from build123d import *

# Parameters (mm, degrees)
CROQUIS1_R              = 55
CROQUIS1_R_2            = 20
SALIENTE_EXTRUIR1_DEPTH = 10
CROQUIS2_R              = 6
CROQUIS2_R_2            = 20
SALIENTE_EXTRUIR2_DEPTH = 20
CROQUIS3_R              = 6
CORTAR_EXTRUIR2_DEPTH   = 81.311892021
CROQUIS4_R              = 4.75
SALIENTE_EXTRUIR3_DEPTH = 5
MATRIZC1_COUNT          = 4
CROQUIS5_R              = 4
CORTAR_EXTRUIR3_DEPTH   = 2.5
MATRIZC2_COUNT          = 6


with BuildPart() as part:
    # Croquis1 → Saliente-Extruir1 (new body)
    with BuildSketch(Plane.XY):
        Circle(CROQUIS1_R)
        Circle(CROQUIS1_R_2, mode=Mode.SUBTRACT)
    extrude(amount=SALIENTE_EXTRUIR1_DEPTH)

    # Croquis2 → Saliente-Extruir2 (add)
    # profile 1 of 7: a face of its own
    with BuildSketch(Plane.XY):
        with Locations((17.368749874, 30.386288484)):
            Circle(CROQUIS2_R)
    # profile 2 of 7: a face of its own
    with BuildSketch(Plane.XY):
        with Locations((35.570236927, 0.06310586)):
            Circle(CROQUIS2_R)
    # profile 3 of 7: a face of its own
    with BuildSketch(Plane.XY):
        with Locations((18.410333978, -30.861435627)):
            Circle(CROQUIS2_R)
    # profile 4 of 7: a face of its own
    with BuildSketch(Plane.XY):
        with Locations((-16.951056024, -31.462794489)):
            Circle(CROQUIS2_R)
    # profile 5 of 7: a face of its own
    with BuildSketch(Plane.XY):
        with Locations((-35.152543077, -1.139611866)):
            Circle(CROQUIS2_R)
    # profile 6 of 7: a face of its own
    with BuildSketch(Plane.XY):
        with Locations((-17.992640128, 29.784929621)):
            Circle(CROQUIS2_R)
    # profile 7 of 7: a face of its own
    with BuildSketch(Plane.XY):
        with BuildLine():
            ThreePointArc((-27.174096814, 22.058296905), (-30.772867756, 16.67424991), (-33.318098438, 10.719343099))
            ThreePointArc((-33.318098438, 10.719343099), (-23.158844078, -0.750787602), (-32.553845663, -12.8548486))
            ThreePointArc((-32.553845663, -12.8548486), (-29.724252158, -18.478875336), (-25.932896476, -23.504996924))
            ThreePointArc((-25.932896476, -23.504996924), (-11.259372102, -20.898480308), (-5.36472656, -34.58640931))
            ThreePointArc((-5.36472656, -34.58640931), (0.788104907, -34.991125884), (6.916475444, -34.309799875))
            ThreePointArc((6.916475444, -34.309799875), (12.262561294, -20.555859902), (26.90508267, -22.385632145))
            ThreePointArc((26.90508267, -22.385632145), (30.429526117, -17.292886986), (33.001146459, -11.658659117))
            ThreePointArc((33.001146459, -11.658659117), (23.570255812, 0.041816456), (32.959571133, 11.775681328))
            ThreePointArc((32.959571133, 11.775681328), (30.28541045, 17.544056369), (26.611824153, 22.733473454))
            ThreePointArc((26.611824153, 22.733473454), (11.413749917, 19.968132432), (6.083961325, 34.467164296))
            ThreePointArc((6.083961325, 34.467164296), (-0.405697858, 34.997648625), (-6.881315891, 34.316868907))
            ThreePointArc((-6.881315891, 34.316868907), (-11.787864219, 19.513573531), (-27.174096814, 22.058296905))
        make_face()
        Circle(CROQUIS2_R_2, mode=Mode.SUBTRACT)
    extrude(amount=SALIENTE_EXTRUIR2_DEPTH)

    # Croquis3 → Cortar-Extruir2 (cut, through all)
    with BuildSketch(Plane.XY.offset(20)):
        with Locations((-17.992640128, 29.784929621)):
            Circle(CROQUIS3_R)
        with Locations((-35.152543077, -1.139611866)):
            Circle(CROQUIS3_R)
        with Locations((-16.951056024, -31.462794489)):
            Circle(CROQUIS3_R)
        with Locations((18.410333978, -30.861435627)):
            Circle(CROQUIS3_R)
        with Locations((35.570236927, 0.06310586)):
            Circle(CROQUIS3_R)
        with Locations((17.368749874, 30.386288484)):
            Circle(CROQUIS3_R)
    extrude(amount=-CORTAR_EXTRUIR2_DEPTH, mode=Mode.SUBTRACT)

    # Croquis4 → Saliente-Extruir3 (add, symmetric)
    with BuildSketch(Plane(origin=(0, 55, 0), x_dir=(1, 0, 0), z_dir=(0, 1, 0))):
        with Locations(Location((0, -5.001814487, 0), (0, 0, 90))):
            Circle(CROQUIS4_R)
    saliente_extruir3 = extrude(amount=SALIENTE_EXTRUIR3_DEPTH, both=True)

    # MatrizC1: Saliente-Extruir3 ×4 about axis
    matrizc1_axis = Axis((0, 0, 0), (0, 0, 1))
    for i in range(1, MATRIZC1_COUNT):
        add(saliente_extruir3.rotate(matrizc1_axis, i * 360 / MATRIZC1_COUNT))

    # Croquis5 → Cortar-Extruir3 (cut, symmetric)
    with BuildSketch(Plane(origin=(0, 35, 0), x_dir=(1, 0, 0), z_dir=(0, 1, 0))):
        with Locations(Location((0, -15.307164254, 0), (0, 0, 270))):
            Circle(CROQUIS5_R)
    cortar_extruir3 = extrude(amount=CORTAR_EXTRUIR3_DEPTH, both=True, mode=Mode.SUBTRACT)

    # MatrizC2: Cortar-Extruir3 ×6 about axis
    matrizc2_axis = Axis((0, 0, 0), (0, 0, 1))
    for i in range(1, MATRIZC2_COUNT):
        add(cortar_extruir3.rotate(matrizc2_axis, i * 360 / MATRIZC2_COUNT), mode=Mode.SUBTRACT)


solid = part.part
Geometry: final body of the model. Coordinates: model frame, mm. A direction names the side the tool comes from. Coordinates: 2 decimals unless noted, no trailing zeros. Order: outer loops, then holes, each group sorted by start corner. A loop starts at its lowest first (then second) coordinate and runs counter-clockwise, first axis right, second up. Notation, with made-up numbers: (64.25, 10) - (78.25, 10) arc R16 cw to (78.25, 34) - close; hole circle Ø1 at (6.25, 30.5). An arc over 180 degrees is marked (long way). Use one line per item in the form item = value.
1) Section B-B (z = 4.5). Return loops of the section in (x, y).
Solutions:
outline = (-60, -4.72) - (-54.8, -4.72) arc R55 ccw to (-4.72, -54.8) - (-4.72, -60) - (4.72, -60) - (4.72, -54.8) arc R55 ccw to (54.8, -4.72) - (60, -4.72) - (60, 4.72) - (54.8, 4.72) arc R55 ccw to (4.72, 54.8) - (4.72, 60) - (-4.72, 60) - (-4.72, 54.8) arc R55 ccw to (-54.8, 4.72) - (-60, 4.72) - close; hole circle Ø12 at (-35.15, -1.14); hole circle Ø12 at (-17.99, 29.78); hole circle Ø12 at (-16.95, -31.46); hole circle Ø40 at (0, 0); hole circle Ø12 at (17.37, 30.39); hole circle Ø12 at (18.41, -30.86); hole circle Ø12 at (35.57, 0.06)
2) Section D-D (x = -45). Return loops of the section in (y, z).
Solutions:
outline = (-31.62, 0) - (31.62, 0) - (31.62, 10) - (-31.62, 10) - close
3) Set-up query: faces 1 (the face through (1.427, -57.433, 0.471)), 2 (the face through (28.118, -16.298, 15.251)), 3 (the face through (57.434, 1.427, 0.471)), 4 (the face through (12.073, -20.672, 14.93)), 5 (the face through (-23.17, -0.52, 14.93)). Return all of +Z, -Z, +X, -X, +Y, -Y with unobstructed straight access to the full face (end or side cutting, diameter ignored); none if empty.
Solutions:
face_1 = -Y
face_2 = none
face_3 = +X
face_4 = +Z
face_5 = +Z, -X
4) Ray query, L1, parallel to X at y = -4.5, z = 8; L2, parallel to Y at x = 0, z = 14; L3, parallel to X at y = 33, z = 8.75. Return the intervals inside material, ascending.
Solutions:
L1 = -54.82 to -40.12, -30.18 to -19.49, 19.49 to 31.67, 39.47 to 54.82
L2 = -32.5 to -20, 20 to 32.5
L3 = -44 to -23.06, -12.93 to 11.97, 22.77 to 44
5) Mould query, pull axis Y, two halves, no side actions, for faces 6 (the face through (-57.434, -1.427, 0.471)), 7 (the face through (32.22, 13.67, 14.93)), 8 (the face through (29.33, 16.73, 11.31)). Classes: +Y half, -Y half, draft (parallel to the pull), parting line (faces both ways), or undercut.
Solutions:
face_6 = parting line
face_7 = +Y half
face_8 = undercut
6) Section C-C (x = -16.5). Return loops of the section in (y, z).
Solutions:
outline = (-52.47, 0) - (-37.45, 0) - (-37.45, 10) - (-52.47, 10) - close; (-25.48, 0) - (-11.3, 0) - (-11.3, 20) - (-19.47, 20) - (-19.47, 10) - (-25.48, 10) - close; (11.3, 0) - (23.97, 0) - (23.97, 10) - (17.88, 10) - (17.88, 20) - (11.3, 20) - close; (35.6, 0) - (52.47, 0) - (52.47, 10) - (35.6, 10) - close
7) Section A-A (x = 0). Return loops of the section in (y, z), then the cut area to 4 significant figures.
Solutions:
outline = (-60, 0.25) - (-55, 0.25) - (-55, 0) - (-20, 0) - (-20, 20) - (-35, 20) - (-35, 19.31) - (-32.5, 19.31) - (-32.5, 11.31) - (-35, 11.31) - (-35, 10) - (-55, 10) - (-55, 9.75) - (-60, 9.75) - close; (20, 0) - (55, 0) - (55, 0.25) - (60, 0.25) - (60, 9.75) - (55, 9.75) - (55, 10) - (35, 10) - (35, 11.31) - (32.5, 11.31) - (32.5, 19.31) - (35, 19.31) - (35, 20) - (20, 20) - close
area = 1,055 mm^2
8) Pin query (flat end, axial travel): pin 1 (1 mm diameter, centred on y = 6, z = 9, fed in from +X); pin 2 (12 mm diameter, centred on x = 24, z = 2, fed in from +Y); pin 3 (6.5 mm diameter, centred on x = -1, z = 17, fed in from +Y); pin 4 (15.5 mm diameter, centred on x = -17.99, y = 29.78, fed in from -Z). Return the tip coordinate at first contact, or that it passes through.
Solutions:
pin_1 = 54.72
pin_2 = 51.97
pin_3 = 35
pin_4 = 0
